Source: CAD feature listing. Evaluate the final solid. Frame: model axes, mm. A direction names the side the tool comes from. Give positions to 0.01 mm unless a question says otherwise; leave off trailing zeros. Loops run counter-clockwise (first coordinate to the right, second up) from the corner with the lowest first, then second, coordinate; pieces in that order, holes last. Notation, with made-up numbers: M 22.5,87 L 61.5,87 A30 ccw 61.5,125 Z; hole C 22.25,19.5 d10. An arc over 180 degrees is marked long. Answer in a Markdown table with one row per item.
```python
from build123d import *

# Parameters (mm, degrees)
F0_W        = 2
F0_H        = 7.85
F0_H_2      = 5.8
F1_DEPTH    = 9.6
F2_T1_DEPTH = 14.5
F3_R        = 0.7
F4_R        = 5


# Not quite as in the source:
# - a fillet or chamfer that OpenCascade refuses, or shapes differently, is made with other operations: its cross-section is extruded or revolved along the edge and cut away or added


with BuildPart() as f1:
    # F0 (on Top) → F1 (new body)
    with BuildSketch(Plane.XY):
        Polygon((-15, 0), (0, 0), (14.1413274131, 16.8529777486), (35.8070979794, 20.6732376573), (35.4077071707, 22.9382954892), (31.9608800352, 22.3305268674), (30.0897453045, 22.0005953298), (23.8854564605, 20.9066118105), (21.9158409545, 20.5593154552), (12.9175229748, 18.9726692144), (-1.0725076138, 2.3), (-5.8, 2.3), (-7.8, 2.3), (-13, 2.3), (-15, 2.3), align=None)
        with Locations((-14, 6.225)):
            Rectangle(F0_W, F0_H)
        with Locations((-6.8, 5.2)):
            Rectangle(F0_W, F0_H_2)
        Polygon((30.0897453045, 22.0005953298), (31.9608800352, 22.3305268674), (31.7004077687, 23.8077384969), (31.3183817778, 25.9743155535), (29.4472470471, 25.644384016), align=None)
        Polygon((31.3183817778, 25.9743155535), (31.7004077687, 23.8077384969), (32.7229194348, 23.9880348917), align=None)
        Polygon((21.9158409545, 20.5593154552), (23.8854564605, 20.9066118105), (23.3818767453, 23.7625542943), (21.4122612392, 23.4152579389), (21.655368688, 22.0365270847), align=None)
        Polygon((20.1781570585, 21.7760548182), (21.655368688, 22.0365270847), (21.4122612392, 23.4152579389), (19.9350496097, 23.1547856724), align=None)
    extrude(amount=F1_DEPTH)

    # F2: fillet of radius 5 on 2 edges, made by hand

    # F2_s2 → F2_t1 (cut)
    with BuildSketch(Plane.YZ.offset(-27.5)):
        with BuildLine():
            ThreePointArc((10.15, 4.6), (8.6855339059, 8.1355339059), (5.15, 9.6))
            Line((5.15, 9.6), (10.15, 9.6))
            Line((10.15, 9.6), (10.15, 4.6))
        make_face()
        with BuildLine():
            ThreePointArc((10.15, 5), (8.6855339059, 1.4644660941), (5.15, 0))
            Line((5.15, 0), (10.15, 0))
            Line((10.15, 0), (10.15, 5))
        make_face()
    extrude(amount=F2_T1_DEPTH, mode=Mode.SUBTRACT)

    # F3
    f3_edges = [f1.edges().sort_by_distance(p)[0] for p in [
        (-13, 2.3, 4.8),
        (-7.8, 2.3, 4.8),
        (-5.8, 2.3, 4.8),
        (-15, 0, 4.8),
        (35.407707, 22.938295, 4.8),
        (35.807098, 20.673238, 4.8),
    ]]
    fillet(f3_edges, radius=F3_R)

    # F4
    f4_edges = [f1.edges().sort_by_distance(p)[0] for p in [
        (0, 0, 4.8),
        (12.917523, 18.972669, 4.8),
        (14.141327, 16.852978, 4.8),
        (-1.072508, 2.3, 4.8),
    ]]
    fillet(f4_edges, radius=F4_R)


solid = f1.part
```
Q1. Contact query for flat-ended pins moving along their axis: pin 1 Ø3 at (y, z) = (15, 1.5) entering from +X; pin 2 Ø5 at (x, z) = (10, 6) entering from -Y; pin 3 Ø5.5 at (y, z) = (5, 7) entering from +X; pin 4 Ø5 at (y, z) = (11.5, 6.5) entering from -X. Output: stop coordinate, or through.
Values follow:
| item | result |
|---|---|
| pin 1 | x = 14.18 |
| pin 2 | y = 8.94 |
| pin 3 | x = 6.5 |
| pin 4 | x = -15 |
Q2. Reachability of faces 1 (the flat face through (21.784, 21.308, 4.733)), 2 (the cylindrical face through (-14.01, 8.65, 8.17)), 3 (the flat face through (6.17, 10.93, 4.73)), 4 (the flat face through (18.363, 19.933, 4.733)) from +Z, -Z, +X, -X, +Y, -Y: full face, straight path, thin tool, end or side. Return the list, or none.
Values follow:
| item | result |
|---|---|
| face 1 | +Z, -Z |
| face 2 | +Z, -X, +Y |
| face 3 | +Z, -Z, +Y |
| face 4 | +Z, -Z, -X |
Q3. Mould query, pull axis X, two halves, no side actions, for faces 5 (the flat face through (10, 13, 0)), 6 (the flat face through (-15, 5, 5)), 7 (the flat face through (31.832, 23.059, 4.733)). Classes: +X half, -X half, draft (parallel to the pull), parting line (faces both ways), or undercut.
Values follow:
| item | result |
|---|---|
| face 5 | draft |
| face 6 | -X half |
| face 7 | undercut |
Q4. Ray query, probe 1 along X at (y, z) = (6.75, 7.5); probe 2 along X at (y, z) = (5.75, 9); probe 3 along Y at (x, z) = (-7, 7.25). Return the intervals inside material, ascending. Write a range as from..to.
Values follow:
| item | result |
|---|---|
| probe 1 | -15..-13, -7.8..-5.8, 2.66..5.66 |
| probe 2 | -15..-13, -7.8..-5.8, 1.82..4.82 |
| probe 3 | 0..8.1 |
Q5. Section query A-A (x = -4). Output: boundary loops of the cut face in (y, z).
Values follow:
| item | result |
|---|---|
| outline | M 0,0 L 2.3,0 L 2.3,9.6 L 0,9.6 Z |
Q6. Section query B-B (y = 14.5). Output: boundary loops of the cut face in (x, z).
Values follow:
| item | result |
|---|---|
| outline | M 9.16,0 L 12.17,0 L 12.17,9.6 L 9.16,9.6 Z |
